Verification items for this drawing (mm, ordinates from the low corner). Round coordinates to 2 decimals unless told otherwise and drop trailing zeros. Order: outer loops, then holes, each group sorted by start corner. A loop starts at its lowest first (then second) coordinate and runs counter-clockwise, first axis right, second up. Notation, with made-up numbers: (67, 34.25) -> (99, 34.25) arc R10 ccw to (99, 51.25) -> close; hole circle Ø1 at (-11.75, 26). An arc over 180 degrees is marked (long way). Answer in a Markdown table with one row per item. Add a question column.
1. Material ranges on L1, parallel to X at y = 0.6, z = 38.6; L2, parallel to Z at x = 59.1, y = 0.65; L3, parallel to X at y = 0.45, z = 12.5, recorded low to high. Write a range as from..to.
2. Sectioned sample at A-A, the plane x = 59.1. Record the boundary of the cut face in (y, z), then the cut area to 3 significant figures.
3. Sectioned sample at B-B, the plane z = 38.6. Record the boundary of the cut face in (x, y).
4. Sectioned sample at C-C, the plane y = 0.95. Record the boundary of the cut face in (x, z), then the cut area to 3 significant figures.
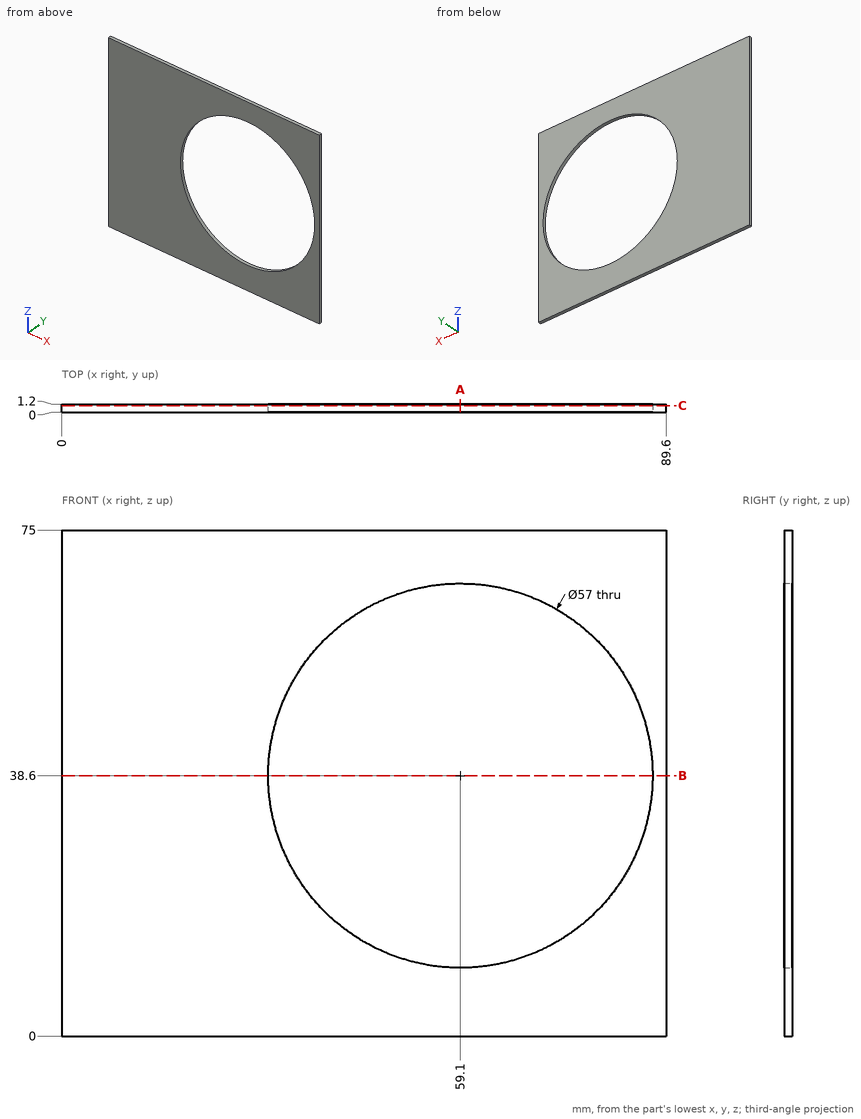
Answer key:
| question | item | result |
|---|---|---|
| 1 | L1 | x = 0..30.6, 87.6..89.6 |
| 1 | L2 | z = 0..10.1, 67.1..75 |
| 1 | L3 | x = 0..47.65, 70.55..89.6 |
| 2 | outline | (0, 0) -> (1.2, 0) -> (1.2, 10.1) -> (0, 10.1) -> close; (0, 67.1) -> (1.2, 67.1) -> (1.2, 75) -> (0, 75) -> close |
| 2 | area | 21.6 mm² |
| 3 | outline | (0, 0) -> (30.6, 0) -> (30.6, 1.2) -> (0, 1.2) -> close; (87.6, 0) -> (89.6, 0) -> (89.6, 1.2) -> (87.6, 1.2) -> close |
| 4 | outline | (0, 0) -> (89.6, 0) -> (89.6, 75) -> (0, 75) -> close; hole circle Ø57 at (59.1, 38.6) |
| 4 | area | 4,170 mm² |
